Autodesk Inventor part; units mm, degrees
ref_plane "YZ Plane" through (0, 0, 0) normal (1, 0, 0) x (0, 1, 0)
ref_plane "XZ Plane" through (0, 0, 0) normal (0, 1, 0) x (-1, 0, 0)
ref_plane "XY Plane" through (0, 0, 0) normal (0, 0, 1) x (1, 0, 0)
sketch "Szkic1" plane through (0, 0, 0) normal (0, 1, 0) x (-1, 0, 0)
  line L0 (0, 0) -> (0, 17.3)
  line L1 (0, 17.3) -> (15, 17.3)
  line L2 (15, 17.3) -> (15, 0)
  line L3 (15, 0) -> (0, 0)
  line L4 (0, 0) -> (0, 4.25)
  line L5 (0, 4.25) -> (-1.5, 4.25)
  line L6 (-1.5, 4.25) -> (16.5, 4.25)
  circle A0 centre (-1.5, 4.25) radius 4.25
  circle A1 centre (16.5, 4.25) radius 4.25
  circle A2 centre (-1.5, 4.25) radius 1.5
  circle A3 centre (16.5, 4.25) radius 1.5
  line L7 (15, 2.75) -> (16.5, 2.75)
  line L8 (16.5, 5.75) -> (15, 5.75)
  line L9 (0, 2.75) -> (-1.5, 2.75)
  line L10 (-1.5, 5.75) -> (0, 5.75)
  dimension "d0" = 17.3
  dimension "d1" = 15
  dimension "d2" = 4.25
  dimension "d3" = 1.5
  dimension "d4" = 18
extrude "Wyciągnięcie proste1" add sketch "Szkic1" along normal blind 11.5 contours L0 L6 A0 | L0 A0 L10 A2 L9 | L0 A0 L6 | A0 L6 A1 L2 L3 L0 | A0 L0 L1 L2 A1 L6 | A1 L2 L6 | L6 L2 A1 | A1 L2 L7 A3 L8
sketch "Szkic2" plane through (0, 0, 0) normal (0, 0, -1) x (-1, 0, 0)
  line L0 (15, 0) -> (15, 11.5)
  line L1 (15, 0) -> (13.5, 0)
  line L2 (0, 0) -> (15, 0)
  line L3 (13.5, 0) -> (13.5, 10)
  line L4 (0, 11.5) -> (15, 11.5)
  line L5 (13.5, 10) -> (1.5, 10)
  line L6 (1.5, 10) -> (1.5, 0)
  dimension "d7" = 1.5
  dimension "d8" = 10
  dimension "d9" = 12
extrude "Wyciągnięcie proste2" cut sketch "Szkic2" against normal blind 20
sketch "Szkic3" plane through (0, 11.5, 0) normal (0, 1, 0) x (1, 0, 0)
  line L0 (0, -17.3) -> (0, -8.2265)
  line L1 (0, -8.8866) -> (6.1207, -8.8866)
  line L2 (6.1207, -8.8866) -> (6.1207, 0)
  line L3 (6.1207, 0) -> (0, 0)
  line L4 (0, 0) -> (0, -8.8866)
  line L5 (-15, -8.2265) -> (-15, -17.3)
  line L6 (-15, -8.8866) -> (-15, 0.446)
  line L7 (-15, 0.446) -> (-21.7347, 0.446)
  line L8 (-21.7347, 0.446) -> (-21.7347, -8.8866)
  line L9 (-21.7347, -8.8866) -> (-15, -8.8866)
extrude "Wyciągnięcie proste3" cut sketch "Szkic3" against normal blind 7
properties part number "przedluzone_mocowanie"
Could you check a few things on this model? Use its own coordinates, in mm. A direction names the side the tool comes from. Give positions to 0.01 mm unless a question says otherwise; leave off trailing zeros. Loops run counter-clockwise (first coordinate to the right, second up) from the corner with the lowest first, then second, coordinate; pieces in that order, holes last. Notation, with made-up numbers: (69.25, 39.5) -> (105.25, 39.5) arc R20 ccw to (105.25, 74.5) -> close; hole circle Ø3 at (79, -11). An arc over 180 degrees is marked (long way). Answer as CSV lines item,"result". Start each with the question number.
(1) We'd pull the mould along X, two halves only. Please class faces 1 (the cylindrical face through (3, 2.2, 4.2)), 2 (the flat face through (1, 0, 7)): released by +X, released by -X, zero draft, split by the parting line, or undercut.
(2) I need wall thicknesses on probe 1 along X at (y, z) = (5.25, 14.75); probe 2 along X at (y, z) = (2, 3); probe 3 along Z at (x, y) = (1, 1.25). Which ranges of each line are inside material? Lowest first, please.
(3) I'm going to push flat-ended pins straight in: pin 1 Ø3.5 at (x, z) = (-7, 9.5) entering from -Y; pin 2 Ø1.5 at (y, z) = (5.5, 3) entering from -X; pin 3 Ø3 at (x, z) = (-18, 3) entering from +Y; pin 4 Ø1.5 at (x, z) = (-16, 4) entering from +Y (3 decimals). Where does each tip first touch, or does it pass through?
(4) If we section it at D-D on z = 2: Write out the boundary of the cut face in (x, y).
(5) If we section it at B-B on z = 14: Write out the boundary of the cut face in (x, y).
(6) Which directions (+Z, -Z, +X, -X, +Y, -Y) give clear straight access to the entire face, cutting with the end or side of a thin tool? Please do faces 3 (the flat face through (-16, 2, 2.75)), 4 (the flat face through (-7.5, 10.4, 17.3)), 5 (the flat face through (-19, 4.5, 4)), 6 (the flat face through (3.5, 4.5, 4.2)), 7 (the flat face through (-13.5, 5, 9)).
(7) If we section it at C-C on x = -7.5: Write out the boundary of the cut face in (y, z), then the cut area to 4 significant figures.
(8) If we section it at A-A on z = 4.25: Write out the boundary of the cut face in (x, y), then the cut area to 4 significant figures.
Computed:
1,face 1,"undercut"
1,face 2,"zero draft"
2,probe 1,"x = -15 to -13.5, -1.5 to 0"
2,probe 2,"x = -20.56 to -17.33, -15 to -13.5, -1.5 to 0, 2.33 to 5.56"
2,probe 3,"z = 0.03 to 2.75, 5.75 to 8.47"
3,pin 1,"stops at y = 10"
3,pin 2,"stops at x = -15"
3,pin 3,"stops at y = 4.5"
3,pin 4,"passes through"
4,outline,"(-20.11, 0) -> (-13.5, 0) -> (-13.5, 10) -> (-1.5, 10) -> (-1.5, 0) -> (5.11, 0) -> (5.11, 4.5) -> (0, 4.5) -> (0, 11.5) -> (-15, 11.5) -> (-15, 4.5) -> (-20.11, 4.5) -> close"
5,outline,"(-15, 0) -> (-13.5, 0) -> (-13.5, 10) -> (-1.5, 10) -> (-1.5, 0) -> (0, 0) -> (0, 11.5) -> (-15, 11.5) -> close"
6,face 3,"+Y, -Y"
6,face 4,"+Z, +X, -X, +Y, -Y"
6,face 5,"+Z, -Z, -X, +Y"
6,face 6,"+Z, -Z, +X, +Y"
6,face 7,"+Z, -Z, -Y"
7,outline,"(10, 0) -> (11.5, 0) -> (11.5, 17.3) -> (10, 17.3) -> close"
7,area,"25.95 mm2"
8,outline,"(-20.75, 0) -> (-18, 0) -> (-18, 4.5) -> (-20.75, 4.5) -> close; (-15, 0) -> (-13.5, 0) -> (-13.5, 10) -> (-1.5, 10) -> (-1.5, 0) -> (0, 0) -> (0, 11.5) -> (-15, 11.5) -> close; (3, 0) -> (5.75, 0) -> (5.75, 4.5) -> (3, 4.5) -> close"
8,area,"77.25 mm2"
